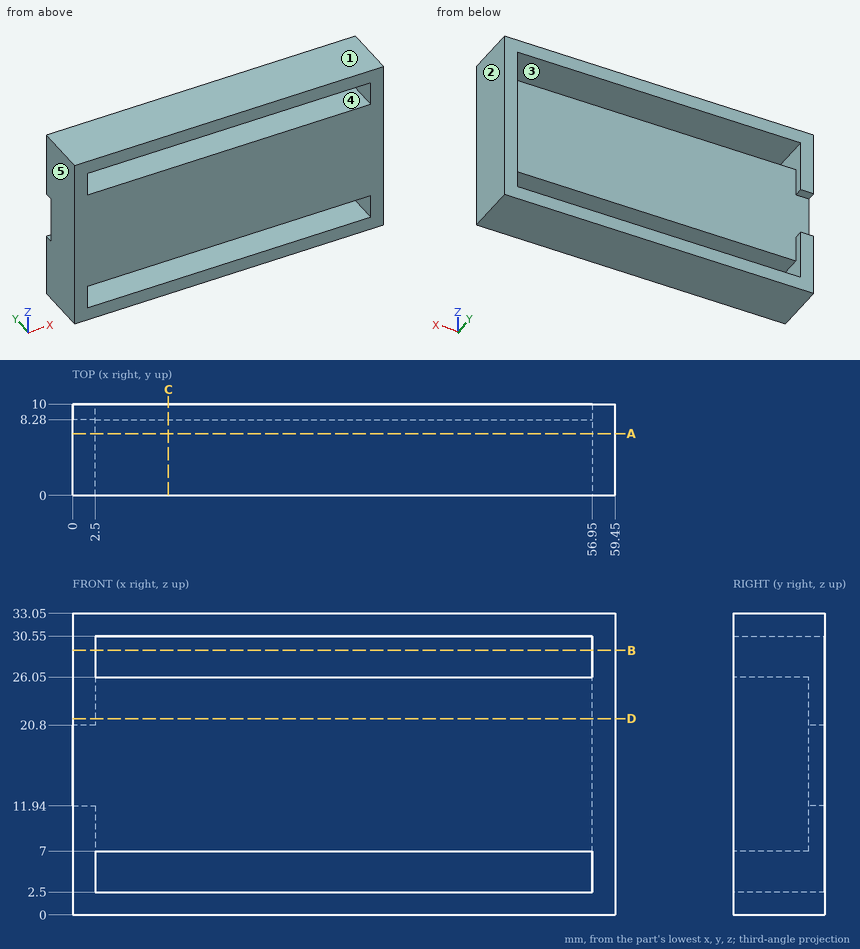
Verification items for this drawing (mm, ordinates from the low corner). A direction names the side the tool comes from. Coordinates: 2 decimals unless noted, no trailing zeros. Write each loop counter-clockwise with the first axis right and the second up, starting at its lowest first coordinate (ties: lowest second). Pieces come first, ordered by that corner, then holes. Notation, with made-up numbers: M 48,83.5 L 93,83.5 A25 cw 93,109.5 Z; hole C 40,85 d4. An arc over 180 degrees is marked long. Use one line per item in the form item = value. Start each with the question number.
1) Set-up check for the marked faces 4 and 5: record each of +Z, -Z, +X, -X, +Y, -Y from which the full face is reachable in a straight line by a thin tool's end or side.
2) Section check A-A on y = 6.75. Enter the section's corners in (x, z), and give its area (3 significant figures).
3) Thickness scan on probe 1 along Z at (x, y) = (29.5, 6); probe 2 along X at (y, z) = (4.75, 6); probe 3 along Z at (x, y) = (27, 9). Record the ranges inside material, lowest first. Write a range as from..to.
4) Section check D-D on z = 21.5. Enter the section's corners in (x, y), and give its area (3 significant figures).
5) Section check C-C on x = 10.5. Enter the section's corners in (y, z), and give its area (3 significant figures).
6) Go/stop test with a flat-tipped pin: pin 1 Ø8 at (x, z) = (28, 13) entering from +Y. Record where the tip stops, or that it passes through.
7) Release check for a two-part mould opening along X. For the marked faces 1, 2 and 3 record: pulls with the +X half, pulls with the -X half, needs draft (parallel to the pull), parting line crosses it, or undercut.
8) Section check B-B on z = 29. Enter the section's corners in (x, y), and give its area (3 significant figures).
Responses:
q1.face_4 = +Y, -Y
q1.face_5 = +Z, -Z, -X, +Y, -Y
q2.outline = M 0,0 L 59.45,0 L 59.45,33.05 L 0,33.05 Z; hole M 2.5,2.5 L 56.95,2.5 L 56.95,7 L 2.5,7 Z; hole M 2.5,26.05 L 56.95,26.05 L 56.95,30.55 L 2.5,30.55 Z
q2.area = 1,470 mm2
q3.probe_1 = 0..2.5, 7..26.05, 30.55..33.05
q3.probe_2 = 0..2.5, 56.95..59.45
q3.probe_3 = 0..2.5, 30.55..33.05
q4.outline = M 0,0 L 59.45,0 L 59.45,10 L 56.95,10 L 56.95,8.28 L 2.5,8.28 L 2.5,10 L 0,10 Z
q4.area = 501 mm2
q5.outline = M 0,0 L 10,0 L 10,2.5 L 0,2.5 Z; M 0,7 L 8.28,7 L 8.28,26.05 L 0,26.05 Z; M 0,30.55 L 10,30.55 L 10,33.05 L 0,33.05 Z
q5.area = 208 mm2
q6.pin_1 = 8.28
q7.face_1 = needs draft
q7.face_2 = pulls with the +X half
q7.face_3 = undercut
q8.outline = M 0,0 L 2.5,0 L 2.5,10 L 0,10 Z; M 56.95,0 L 59.45,0 L 59.45,10 L 56.95,10 Z
q8.area = 50.0 mm2
